from build123d import *

# Parameters (mm, degrees)
SKETCH1_R           = 107.95
SKETCH1_R_2         = 95.25
BOSS_EXTRUDE1_DEPTH = 6.35
SKETCH2_R           = 2.085
SKETCH2_R_2         = 2.413
CUT_EXTRUDE1_DEPTH  = 21.336
SKETCH3_R           = 9.338597003
CUT_EXTRUDE2_DEPTH  = 7.35
SKETCH4_R           = 2.413
CUT_EXTRUDE3_DEPTH  = 6.35


with BuildPart() as part:
    # Sketch1 → Boss-Extrude1 (new body)
    with BuildSketch(Plane.XY):
        with Locations((14.57950887, 23.250008023)):
            Circle(SKETCH1_R)
        with Locations((14.57950887, 23.250008023)):
            Circle(SKETCH1_R_2, mode=Mode.SUBTRACT)
    extrude(amount=BOSS_EXTRUDE1_DEPTH)

    # Sketch2 → Cut-Extrude1 (cut)
    with BuildSketch(Plane(origin=(0, 0, 0), x_dir=(-1, 0, 0), z_dir=(0, 0, -1))):
        with Locations((-104.081912459, 71.332018712)):
            Circle(SKETCH2_R)
        with Locations((-17.690467943, 124.802368575)):
            Circle(SKETCH2_R)
        with Locations((71.811935646, 76.720357886)):
            Circle(SKETCH2_R)
        with Locations((74.922894719, -24.832002665)):
            Circle(SKETCH2_R)
        with Locations((-11.468549797, -78.302352529)):
            Circle(SKETCH2_R)
        with Locations((-100.970953386, -30.22034184)):
            Circle(SKETCH2_R)
        with Locations((4.215773698, 124.891191499)):
            Circle(SKETCH2_R_2)
        with Locations((-114.220260226, 50.557967298)):
            Circle(SKETCH2_R_2)
    extrude(amount=-CUT_EXTRUDE1_DEPTH, mode=Mode.SUBTRACT)

    # Sketch3 → Cut-Extrude2 (cut, through all)
    with BuildSketch(Plane(origin=(0, 0, 0), x_dir=(-1, 0, 0), z_dir=(0, 0, -1))):
        with Locations((-65.924155814, 105.010280384)):
            Circle(SKETCH3_R)
    extrude(amount=-CUT_EXTRUDE2_DEPTH, mode=Mode.SUBTRACT)

    # Sketch4 → Cut-Extrude3 (cut)
    with BuildSketch(Plane.XY.offset(6.35)):
        with Locations((33.116626404, -78.229145041)):
            Circle(SKETCH4_R)
        with Locations((-85.036904703, -4.073226214)):
            Circle(SKETCH4_R)
    extrude(amount=-CUT_EXTRUDE3_DEPTH, mode=Mode.SUBTRACT)


solid = part.part
Work out the finished part from the listing and answer in its coordinate system (mm). Give positions to 0.01 mm unless a question says otherwise; leave off trailing zeros. Order: outer loops, then holes, each group sorted by start corner. A loop starts at its lowest first (then second) coordinate and runs counter-clockwise, first axis right, second up. Notation, with made-up numbers: (7.25, -19.5) -> (17.25, -19.5) arc R28 cw to (17.25, 0.5) -> close; hole circle Ø8 at (-28.5, -34.5). An arc over 180 degrees is marked (long way). Answer as a JSON object with one key per item and string values. Group by question number.
1. Flat-ended cylindrical pins translate along their axes: pin 1 Ø1.5 at (x, z) = (21, 1) entering from -Y; pin 2 Ø3 at (y, z) = (7, 2.5) entering from -X. Find the tip coordinate at first contact, or state that the pin passes through.
2. Section C-C on z = 3.5 is taken. Count the separate pieces of the cut face and the enclosed holes in it, plus the area to 3 significant figures.
3. Section B-B on x = -30.5 is taken. Determine the outline of the cut face in (y, z).
4. Section A-A on y = -54 is taken. Determine the outline of the cut face in (x, z).
5. Consider line 1 along Y through (x, z) = (15.5, 4.75); line 2 along Y through (x, z) = (-70.5, 4.25); line 3 along X through (y, z) = (21, 2.25). Determine where each line is inside the solid, lowest interval first. Write a range as [from, to].
6. The mould has two halves that part along X. Classify faces 1 (the cylindrical face through (-8.822, -82.133, 3.131)), 2 (the flat face through (14.1, -72.2, 6.35)), 3 (the cylindrical face through (-39.47, -55.18, 3.13)): released by +X, released by -X, zero draft, split by the parting line, or undercut.
Result sheet:
{
 "1": {"pin 1": "stops at y = -84.55", "pin 2": "stops at x = -92.36"},
 "2": {"separate pieces": "1", "enclosed holes": "11", "area": "7,790 mm^2"},
 "3": {"outline": "(-74.84, 0) -> (-60.66, 0) -> (-60.66, 6.35) -> (-74.84, 6.35) -> close; (107.16, 0) -> (121.34, 0) -> (121.34, 6.35) -> (107.16, 6.35) -> close"},
 "4": {"outline": "(-60.82, 0) -> (-41.14, 0) -> (-41.14, 6.35) -> (-60.82, 6.35) -> close; (70.3, 0) -> (89.98, 0) -> (89.98, 6.35) -> (70.3, 6.35) -> close"},
 "5": {"line 1": "y = [-84.7, -72], [118.5, 131.2]", "line 2": "y = [-43.19, -19.58], [66.08, 75.1], [78.34, 89.69]", "line 3": "x = [-93.35, -80.64], [109.8, 122.51]"},
 "6": {"face 1": "split by the parting line", "face 2": "zero draft", "face 3": "undercut"}
}
